Autodesk Inventor part; units mm, degrees
ref_plane "YZ Plane" through (0, 0, 0) normal (1, 0, 0) x (0, 1, 0)
ref_plane "XZ Plane" through (0, 0, 0) normal (0, 1, 0) x (-1, 0, 0)
ref_plane "XY Plane" through (0, 0, 0) normal (0, 0, 1) x (1, 0, 0)
sketch "Sketch1" plane through (0, 0, 0) normal (0, 0, 1) x (1, 0, 0)
  line L0 (-25.4, 152.4) -> (25.4, 152.4)
  line L1 (25.4, 152.4) -> (25.4, -152.4)
  line L2 (25.4, -152.4) -> (-25.4, -152.4)
  line L3 (-25.4, -152.4) -> (-25.4, 152.4)
  line L4 (-25.4, 152.4) -> (25.4, -152.4) construction
  line L5 (25.4, 152.4) -> (-25.4, -152.4) construction
  circle A0 centre (-7.9375, -12.7) radius 25.4 construction
  circle A1 centre (-7.9375, -12.7) radius 11.1125
  circle A2 centre (-7.9375, -12.7) radius 38.1 construction
  circle A3 centre (-7.9375, -12.7) radius 50.8 construction
  circle A4 centre (-7.9375, 101.6) radius 25.4 construction
  circle A5 centre (-7.9375, 101.6) radius 11.1125
  circle A6 centre (-7.9375, 101.6) radius 38.1 construction
  circle A7 centre (-7.9375, 101.6) radius 50.8 construction
  point P0 (0, 0)
  dimension "d0" = 50.8
  dimension "d1" = 304.8
  dimension "d3" = 50.8
  dimension "d4" = 22.225
  dimension "d7" = 17.4625
  dimension "d8" = 76.2
  dimension "d9" = 101.6
  dimension "d10" = 50.8
  dimension "d11" = 22.225
  dimension "d12" = 76.2
  dimension "d13" = 101.6
  dimension "d14" = 114.3
  dimension "d15" = 139.7
extrude "Extrusion1" add sketch "Sketch1" along normal blind 6.35
sketch "Sketch2" plane through (0, 0, 6.35) normal (0, 0, 1) x (1, 0, 0)
  line L0 (-25.4, 152.4) -> (-25.4, -152.4) construction
  line L1 (-12.7, -107.95) -> (12.7, -107.95) construction
  line L2 (-25.4, -152.4) -> (25.4, -152.4) construction
  point P0 (0, 0)
  point P1 (-12.7, -146.05)
  point P2 (12.7, -146.05)
  point P3 (0, -107.95)
  dimension "d19" = 25.4
  dimension "d21" = 38.1
  dimension "d22" = 6.35
hole "Hole1" at (-12.7, -107.95, 6.35) at (12.7, -107.95, 6.35) at (-12.7, -146.05, 6.35) at (12.7, -146.05, 6.35) direction (0, 0, -1) diameter 5.1054 end through all
properties part number "GP1-002" material "Aluminum 6061"
Part model, mm, in its own coordinate system. Coordinates: 2 decimals unless noted, no trailing zeros. Loops run counter-clockwise (first coordinate to the right, second up) from the corner with the lowest first, then second, coordinate; pieces in that order, holes last. Notation, with made-up numbers: (-40, -30.5) -> (-13, -30.5) arc R22 ccw to (-13, -19.5) -> close; hole circle Ø7 at (46.25, 65.5). An arc over 180 degrees is marked (long way). Use a Markdown table: item, result. Add a question column.
Item 1: Band-saw the part on A-A on z = 3.5. Give the number of separate pieces and of enclosed holes in the cut face, plus the area to 3 significant figures.
Item 2: Flat gauge pin, fed straight in: P1, Ø6, axis at x = -12.7, y = -107.95, coming from the -Z side. Where does the tip first touch, or does it go through?
Item 3: Probe probe 1 along X at (y, z) = (-146.05, 3); probe 2 along Y at (x, z) = (13, 4); probe 3 along Y at (x, z) = (-14.5, 3.25). List the from-to ranges inside material, lowest first.
Item 4: Band-saw the part on C-C on x = 12.7. Write the cut outline in (y, z), plus the area to 3 significant figures.
Item 5: Band-saw the part on D-D on y = -12.7. Write the cut outline in (x, z) (3 decimals).
Item 6: Band-saw the part on B-B on y = -107.95. Write the cut outline in (x, z).
Item 7: Pull direction X, two halves, no side cores. Call faces 1 (the cylindrical face through (11.933, -148.485, 3.131)), 2 (the cylindrical face through (-12.8, -105.4, 3.1)), 3 (the flat face through (0, 152.4, 3)), 4 (the flat face through (-25.4, -2, 3)): +X half, -X half, draft (parallel to the pull), parting line (faces both ways), or undercut.
Geometry says:
| question | item | result |
|---|---|---|
| 1 | separate pieces | 1 |
| 1 | enclosed holes | 6 |
| 1 | area | 14,600 mm² |
| 2 | P1 | z = 0 |
| 3 | probe 1 | -25.4 to -15.25, -10.15 to 10.15, 15.25 to 25.4 |
| 3 | probe 2 | -152.4 to -148.59, -143.51 to -110.49, -105.41 to 152.4 |
| 3 | probe 3 | -152.4 to -147.86, -144.24 to -109.76, -106.14 to -21.67, -3.73 to 92.63, 110.57 to 152.4 |
| 4 | outline | (-152.4, 0) -> (-148.6, 0) -> (-148.6, 6.35) -> (-152.4, 6.35) -> close; (-143.5, 0) -> (-110.5, 0) -> (-110.5, 6.35) -> (-143.5, 6.35) -> close; (-105.4, 0) -> (152.4, 0) -> (152.4, 6.35) -> (-105.4, 6.35) -> close |
| 4 | area | 1,870 mm² |
| 5 | outline | (-25.4, 0) -> (-19.05, 0) -> (-19.05, 6.35) -> (-25.4, 6.35) -> close; (3.175, 0) -> (25.4, 0) -> (25.4, 6.35) -> (3.175, 6.35) -> close |
| 6 | outline | (-25.4, 0) -> (-15.25, 0) -> (-15.25, 6.35) -> (-25.4, 6.35) -> close; (-10.15, 0) -> (10.15, 0) -> (10.15, 6.35) -> (-10.15, 6.35) -> close; (15.25, 0) -> (25.4, 0) -> (25.4, 6.35) -> (15.25, 6.35) -> close |
| 7 | face 1 | undercut |
| 7 | face 2 | undercut |
| 7 | face 3 | draft |
| 7 | face 4 | -X half |
